Verification items for the finished model (mm, model axes). Face numbers are marked on the shaded views. Coordinates: 2 decimals unless noted, no trailing zeros. Order: outer loops, then holes, each group sorted by start corner. A loop starts at its lowest first (then second) coordinate and runs counter-clockwise, first axis right, second up.
Q1. Cross-section at C-C, the plane z = 4. Count the separate pieces of the cut face and the enclosed holes in it, and give its area (3 significant figures).
Q2. Draft check along Y on the marked faces 1, 2, 3 and 4. Enter one of: pulls with the +Y half, pulls with the -Y half, needs draft (parallel to the pull), parting line crosses it, or undercut.
Q3. Thickness scan on line 1 (Y direction, x = -8, z = 22.5); line 2 (Z direction, x = 17.5, y = -17.5); line 3 (Z direction, x = 20.5, y = 16). Record the ranges inside material, lowest first.
Q4. Cross-section at D-D, the plane x = -14.5. Record the boundary of the cut face in (y, z), and give its area (4 significant figures).
Q5. Depth check by flat-ended pin: P1, Ø2.5, axis at y = -37.5, z = 3, coming from the -X side; P2, Ø3, axis at x = -3.5, y = -20.5, coming from the +Z side; P3, Ø10, axis at x = -14.5, y = 5.5, coming from the +Z side. Enter the tip coordinate at first touch or a pass-through.
Q6. Cross-section at A-A, the plane z = 23.5. Record the boundary of the cut face in (x, y), and give its area (3 significant figures).
Q7. Cross-section at B-B, the plane y = 39. Record the boundary of the cut face in (x, z), and give its area (3 significant figures).
from build123d import *

# Parameters (mm, degrees)
SKETCH1_W            = 55
SKETCH1_H            = 67
BOSS_EXTRUDE1_DEPTH  = 2.5
SKETCH2_W            = 55
SKETCH2_H            = 3
BOSS_EXTRUDE2_DEPTH  = 25
SKETCH3_R            = 5
SKETCH3_R_2          = 3.025
BOSS_EXTRUDE3_DEPTH  = 3
CUT_EXTRUDE1_START   = -2
SKETCH4_R            = 3.025
CUT_EXTRUDE1_DEPTH   = 2
SKETCH5_W            = 5.5
SKETCH5_H            = 11
BOSS_EXTRUDE4_DEPTH  = 5
M4_CLEARANCE_HOLE1_D = 4.8
FILLET3_R            = 2


with BuildPart() as part:
    # Sketch1 → Boss-Extrude1 (new body)
    with BuildSketch(Plane.XY):
        Rectangle(SKETCH1_W, SKETCH1_H)
    extrude(amount=BOSS_EXTRUDE1_DEPTH)

    # Sketch2 → Boss-Extrude2 (add)
    with BuildSketch(Plane.XY.offset(2.5)):
        with Locations((0, 32)):
            Rectangle(SKETCH2_W, SKETCH2_H)
        with Locations((0, -32)):
            Rectangle(SKETCH2_W, SKETCH2_H)
    extrude(amount=BOSS_EXTRUDE2_DEPTH)

    # Sketch3 → Boss-Extrude3 (add)
    # profile 1 of 4: a face of its own
    with BuildSketch(Plane.XY.offset(2.5)):
        with Locations((-2.504, 19.6215)):
            Circle(SKETCH3_R)
        with Locations((-2.504, 19.6215)):
            Circle(SKETCH3_R_2, mode=Mode.SUBTRACT)
    # profile 2 of 4: a face of its own
    with BuildSketch(Plane.XY.offset(2.5)):
        with Locations((16.546, 19.6215)):
            Circle(SKETCH3_R)
        with Locations((16.546, 19.6215)):
            Circle(SKETCH3_R_2, mode=Mode.SUBTRACT)
    # profile 3 of 4: a face of its own
    with BuildSketch(Plane.XY.offset(2.5)):
        with Locations((16.546, -19.6215)):
            Circle(SKETCH3_R)
        with Locations((16.546, -19.6215)):
            Circle(SKETCH3_R_2, mode=Mode.SUBTRACT)
    # profile 4 of 4: a face of its own
    with BuildSketch(Plane.XY.offset(2.5)):
        with Locations((-2.504, -19.6215)):
            Circle(SKETCH3_R)
        with Locations((-2.504, -19.6215)):
            Circle(SKETCH3_R_2, mode=Mode.SUBTRACT)
    extrude(amount=BOSS_EXTRUDE3_DEPTH)

    # Sketch4 → Cut-Extrude1 (cut)
    with BuildSketch(Plane.XY.offset(2.5).offset(CUT_EXTRUDE1_START)):
        with Locations((16.546, -19.6215)):
            Circle(SKETCH4_R)
        with Locations((-2.504, -19.6215)):
            Circle(SKETCH4_R)
        with Locations((16.546, 19.6215)):
            Circle(SKETCH4_R)
        with Locations((-2.504, 19.6215)):
            Circle(SKETCH4_R)
    extrude(amount=CUT_EXTRUDE1_DEPTH, mode=Mode.SUBTRACT)

    # Sketch5 → Boss-Extrude4 (add)
    with BuildSketch(Plane(origin=(0, 0, 0), x_dir=(-1, 0, 0), z_dir=(0, 0, -1))):
        with Locations((-9.75, 39)):
            Rectangle(SKETCH5_W, SKETCH5_H)
        with Locations((-15.25, 39)):
            Rectangle(SKETCH5_W, SKETCH5_H)
    boss_extrude4 = extrude(amount=-BOSS_EXTRUDE4_DEPTH)

    # M4 Clearance Hole1 (through all)
    with Locations(Plane.XY.offset(5)):
        with Locations((12.5, 39)):
            m4_clearance_hole1 = Hole(M4_CLEARANCE_HOLE1_D / 2)

    # Mirror2: Boss-Extrude4, M4 Clearance Hole1 across plane
    add(boss_extrude4.mirror(Plane.ZX))
    add(m4_clearance_hole1.mirror(Plane.ZX), mode=Mode.SUBTRACT)

    # Fillet3
    fillet3_edges = [part.edges().sort_by_distance(p)[0] for p in [
        (7, -44.5, 2.5),
        (18, -44.5, 2.5),
        (18, -33.5, 2.5),
        (7, -33.5, 2.5),
        (18, 44.5, 2.5),
        (7, 44.5, 2.5),
        (7, 33.5, 2.5),
        (18, 33.5, 2.5),
    ]]
    fillet(fillet3_edges, radius=FILLET3_R)


solid = part.part
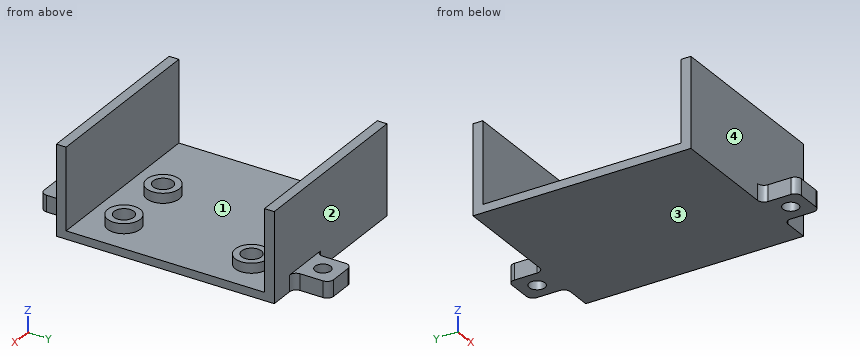
Check values:
1. separate pieces: 6
1. enclosed holes: 6
1. area: 735 mm2
2. face 1: undercut
2. face 2: pulls with the +Y half
2. face 3: needs draft
2. face 4: pulls with the -Y half
3. line 1: y = -33.5 to -30.5, 30.5 to 33.5
3. line 2: z = 0 to 0.5
3. line 3: z = 0 to 2.5
4. outline: (-33.5, 0) - (33.5, 0) - (33.5, 27.5) - (30.5, 27.5) - (30.5, 2.5) - (-30.5, 2.5) - (-30.5, 27.5) - (-33.5, 27.5) - close
4. area: 317.5 mm2
5. P1: stops at x = 7
5. P2: stops at z = 0.5
5. P3: stops at z = 2.5
6. outline: (-27.5, -33.5) - (27.5, -33.5) - (27.5, -30.5) - (-27.5, -30.5) - close; (-27.5, 30.5) - (27.5, 30.5) - (27.5, 33.5) - (-27.5, 33.5) - close
6. area: 330 mm2
7. outline: (7, 0) - (10.1, 0) - (10.1, 5) - (7, 5) - close; (14.9, 0) - (18, 0) - (18, 5) - (14.9, 5) - close
7. area: 31.0 mm2
